The model under review builds one solid part; all positions refer to its coordinate system, in mm. Face numbers are marked on the shaded views. A direction names the side the tool comes from. Round coordinates to 2 decimals unless told otherwise and drop trailing zeros. Write each loop counter-clockwise with the first axis right and the second up, starting at its lowest first coordinate (ties: lowest second). Pieces come first, ordered by that corner, then holes.
Item 1: Add section B-B (y = 14.25). Give the boundary of the cut face in (x, z).
Item 2: To check wall thickness, follow L1, parallel to Z at x = 5, y = 15.5; L2, parallel to Z at x = 34, y = 6; L3, parallel to Y at x = 19, z = -17. State the ranges of each line that lie inside material, in increasing order.
Item 3: Machinability: for the marked faces 4, 5 and 6, which of the approach directions +Z, -Z, +X, -X, +Y, -Y give a long, thin tool a straight path to every point of the face, cutting with its end or side? Answer none if there is none.
Item 4: Draft analysis for pull direction Z (two halves, no side actions). For the marked faces 1, 2 and 3, state which applies: +Z half, -Z half, draft (parallel to the pull), parting line (faces both ways), or undercut.
Item 5: Add section A-A (y = 1.75). Give the boundary of the cut face in (x, z), plus the area to 3 significant figures.
Item 6: Add section C-C (z = -10). Give the boundary of the cut face in (x, y).
Item 7: Add section D-D (x = 37.5). Give the boundary of the cut face in (y, z), plus the area to 3 significant figures.
Item 8: Clearance check with flat-ended pins moving along their axes: pin 1 Ø6.5 at (x, z) = (32, -3) entering from +Y; pin 2 Ø2.5 at (y, z) = (-3, -7) entering from -X; pin 3 Ø1 at (y, z) = (8.5, 37.5) entering from +X; pin 4 Ø1.6 at (y, z) = (6.5, 30.5) entering from +X. State where each tip first meets the part, or that it passes through.
```python
from build123d import *

# Parameters (mm, degrees)
BOSS_EXTRUDE1_DEPTH  = 69.99986
SKETCH2_W            = 23
SKETCH2_H            = 14
CUT_EXTRUDE1_DEPTH   = 2
BOSS_EXTRUDE10_DEPTH = 10
CHAMFER2_SIZE        = 1
SKETCH10_R           = 1.5
CUT_EXTRUDE5_DEPTH   = 90.467972845
SKETCH11_R           = 1.6
CUT_EXTRUDE6_DEPTH   = 78.279501445
CUT_EXTRUDE7_DEPTH   = 14.9


with BuildPart() as part:
    # Sketch1 → Boss-Extrude1 (new body)
    with BuildSketch(Plane.ZY.offset(29.759563114)):
        Polygon((-16.355611523, -2.282836071), (-18.355611523, -2.282836071), (-18.355611523, -4.782836071), (18.644388477, -4.782836071), (18.644388477, -2.282836071), (16.644388477, -2.282836071), (16.644388477, 17.217163929), (19.644388477, 17.217163929), (19.644388477, 10.217163929), (17.644388477, 10.217163929), (17.644388477, 7.617163929), (50.644324477, 7.617163929), (50.644324477, 10.217163929), (48.644324477, 10.217163929), (48.644324477, 17.217163929), (52.144356477, 17.217163929), (52.144356477, -9.782836071), (-19.855643523, -9.782836071), (-19.855643523, 17.217163929), (-16.355611523, 17.217163929), align=None)
    extrude(amount=-BOSS_EXTRUDE1_DEPTH)

    # Sketch2 → Cut-Extrude1 (cut)
    with BuildSketch(Plane(origin=(0, 7.617163929, 0), x_dir=(1, 0, 0), z_dir=(0, 1, 0))):
        with Locations((28.740296886, -27.644388477)):
            Rectangle(SKETCH2_W, SKETCH2_H)
    extrude(amount=-CUT_EXTRUDE1_DEPTH, mode=Mode.SUBTRACT)

    # Sketch9 → Boss-Extrude10 (add)
    with BuildSketch(Plane(origin=(40.240296886, 0, 0), x_dir=(0, 0, -1), z_dir=(1, 0, 0))):
        Polygon((-48.644324477, 17.217163929), (-52.144356477, 17.217163929), (-52.144356477, -9.782836071), (19.855643523, -9.782836071), (19.855643523, 17.217163929), (16.355611523, 17.217163929), (16.355611523, -1.782836071), (-50.644324477, -1.782836071), (-50.644324477, 10.217163929), (-48.644324477, 10.217163929), align=None)
    extrude(amount=BOSS_EXTRUDE10_DEPTH)

    # Chamfer2
    chamfer2_edges = [part.edges().sort_by_distance(p)[0] for p in [
        (-29.759563114, 3.717163929, -19.855643523),
        (-29.759563114, 3.717163929, 52.144356477),
        (50.240296886, 3.717163929, 52.144356477),
        (50.240296886, 3.717163929, -19.855643523),
    ]]
    chamfer(chamfer2_edges, length=CHAMFER2_SIZE)

    # Sketch10 → Cut-Extrude5 (cut, through all)
    with BuildSketch(Plane.XY.offset(52.144356477)):
        with Locations((10.240366886, -7.282836071)):
            Circle(SKETCH10_R)
    extrude(amount=-CUT_EXTRUDE5_DEPTH, mode=Mode.SUBTRACT)

    # Sketch11 → Cut-Extrude6 (cut, through all)
    with BuildSketch(Plane.XZ.offset(9.782836071)):
        with Locations(Location((-12.013114804, 36.144356477, 0), (0, 0, 270))):
            Circle(SKETCH11_R)
        with Locations(Location((32.493848577, -3.855643523, 0), (0, 0, 270))):
            Circle(SKETCH11_R)
    extrude(amount=-CUT_EXTRUDE6_DEPTH, mode=Mode.SUBTRACT)

    # Sketch12 → Cut-Extrude7 (cut)
    with BuildSketch(Plane(origin=(0, 7.617163929, 0), x_dir=(1, 0, 0), z_dir=(0, 1, 0))):
        Polygon((-12.013114804, -32.680254862), (-15.013114804, -34.412305669), (-15.013114804, -37.876407284), (-12.013114804, -39.608458092), (-9.013114804, -37.876407284), (-9.013114804, -34.412305669), align=None)
        Polygon((32.493848577, 7.319745138), (29.493848577, 5.587694331), (29.493848577, 2.123592716), (32.493848577, 0.391541908), (35.493848577, 2.123592716), (35.493848577, 5.587694331), align=None)
    extrude(amount=-CUT_EXTRUDE7_DEPTH, mode=Mode.SUBTRACT)


solid = part.part
```
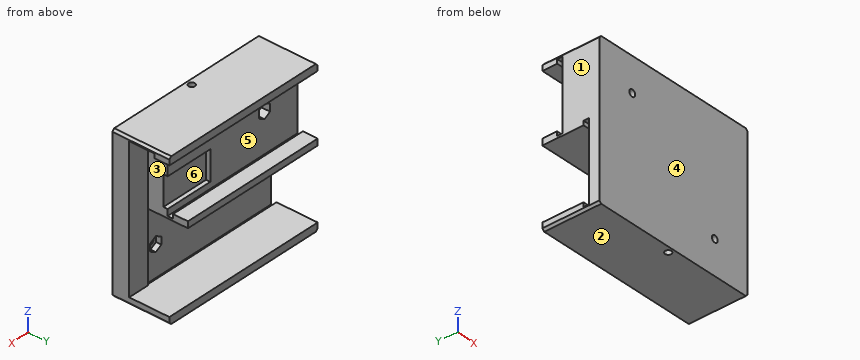
Numbers:
1. outline: (-29.76, -18.86) - (-28.76, -19.86) - (49.24, -19.86) - (50.24, -18.86) - (50.24, -16.36) - (-29.76, -16.36) - close; (-29.76, 16.64) - (40.24, 16.64) - (40.24, 19.64) - (-29.76, 19.64) - close; (-29.76, 48.64) - (50.24, 48.64) - (50.24, 51.14) - (49.24, 52.14) - (-28.76, 52.14) - (-29.76, 51.14) - close
2. L1: z = -19.86 to -16.36, 16.64 to 19.64, 48.64 to 52.14
2. L2: z = -19.86 to -16.36, 16.64 to 20.64, 34.64 to 52.14
2. L3: y = -9.78 to -4.78, -2.28 to 17.22
3. face 4: +Z, -Z, +X, -X, -Y
3. face 5: +X, -X
3. face 6: +X, +Y
4. face 1: draft
4. face 2: -Z half
4. face 3: undercut
5. outline: (-29.76, -18.86) - (-28.76, -19.86) - (49.24, -19.86) - (50.24, -18.86) - (50.24, -16.36) - (-29.76, -16.36) - close; (-29.76, 16.64) - (40.24, 16.64) - (40.24, 50.64) - (50.24, 50.64) - (50.24, 51.14) - (49.24, 52.14) - (-28.76, 52.14) - (-29.76, 51.14) - close; hole (-15.01, 34.41) - (-12.01, 32.68) - (-9.01, 34.41) - (-9.01, 37.88) - (-12.01, 39.61) - (-15.01, 37.88) - close
5. area: 2,750 mm2
6. outline: (-29.76, -9.78) - (50.24, -9.78) - (50.24, -1.78) - (40.24, -1.78) - (40.24, -4.78) - (-29.76, -4.78) - close; hole circle Ø3 at (10.24, -7.28)
7. outline: (-9.78, -19.86) - (17.22, -19.86) - (17.22, -16.36) - (-2.28, -16.36) - (-2.28, -18.36) - (-4.78, -18.36) - (-4.78, 18.64) - (-2.28, 18.64) - (-2.28, 16.64) - (17.22, 16.64) - (17.22, 19.64) - (10.22, 19.64) - (10.22, 17.64) - (7.62, 17.64) - (7.62, 20.64) - (5.62, 20.64) - (5.62, 34.64) - (7.62, 34.64) - (7.62, 50.64) - (10.22, 50.64) - (10.22, 48.64) - (17.22, 48.64) - (17.22, 52.14) - (-9.78, 52.14) - close
7. area: 891 mm2
8. pin 1: stops at y = -4.78
8. pin 2: stops at x = 40.24
8. pin 3: passes through
8. pin 4: stops at x = 17.24
